The listing builds one solid part. Answer for the finished solid, in the listing's coordinates (mm). Give positions to 0.01 mm unless a question says otherwise; leave off trailing zeros. Order: outer loops, then holes, each group sorted by start corner. A loop starts at its lowest first (then second) coordinate and runs counter-clockwise, first axis right, second up. Notation, with made-up numbers: (1.25, 71) - (54.25, 71) arc R16 cw to (54.25, 85) - close; hole circle Ø2 at (-31, 45.5). An arc over 180 degrees is marked (long way). Answer in a Markdown table with one row per item.
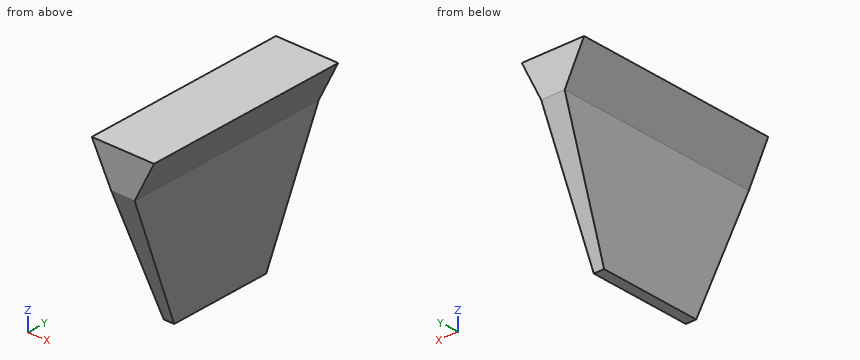
from build123d import *

# Parameters (mm, degrees)
BOSS_EXTRUDE1_DEPTH = 80
SKETCH2_W           = 9.06
SKETCH2_H           = 80
BOSS_EXTRUDE2_DEPTH = 50
CUT_EXTRUDE1_DEPTH  = 105.399039741
CUT_EXTRUDE2_DEPTH  = 106.848049103


with BuildPart() as part:
    # Sketch1 → Boss-Extrude1 (new body)
    with BuildSketch(Plane(origin=(0, 0, 0), x_dir=(1, 0, 0), z_dir=(0, 1, 0))):
        Polygon((-24.06, 0), (-16.56, 14.999429989), (-7.5, 14.999429989), (0, 0), align=None)
    extrude(amount=BOSS_EXTRUDE1_DEPTH)

    # Sketch2 → Boss-Extrude2 (add)
    with BuildSketch(Plane(origin=(0, 0, -14.999429989), x_dir=(-1, 0, 0), z_dir=(0, 0, -1))):
        with Locations((12.03, 40)):
            Rectangle(SKETCH2_W, SKETCH2_H)
    extrude(amount=BOSS_EXTRUDE2_DEPTH)

    # Sketch3 → Cut-Extrude1 (cut, through all)
    with BuildSketch(Plane.ZY.offset(16.56)):
        Polygon((-14.999429989, 80), (-64.999429989, 60), (-64.999429989, 80), align=None)
        Polygon((-64.999429989, 0), (-64.999429989, 20), (-14.999429989, 0), align=None)
    extrude(amount=-CUT_EXTRUDE1_DEPTH, mode=Mode.SUBTRACT)

    # Sketch7 → Cut-Extrude2 (cut, through all)
    with BuildSketch(Plane(origin=(0, 80, 0), x_dir=(1, 0, 0), z_dir=(0, 1, 0))):
        Polygon((-16.56, 14.999429989), (-14.03, 64.999429989), (-16.56, 64.999429989), align=None)
        Polygon((-7.5, 14.999429989), (-7.5, 64.999429989), (-10.03, 64.999429989), align=None)
    extrude(amount=-CUT_EXTRUDE2_DEPTH, mode=Mode.SUBTRACT)


solid = part.part
Item 1: Find section D-D on x = -22. Write down the section's boundary in (y, z).
Answer block:
| item | result |
|---|---|
| outline | (0, -4.12) - (80, -4.12) - (80, 0) - (0, 0) - close |
Item 2: Consider line 1 (Z direction, x = -18, y = 34); line 2 (X direction, y = 38, z = -16); line 3 (X direction, y = 26, z = -37). Determine where each line is inside the solid, lowest interval first.
Answer block:
| item | result |
|---|---|
| line 1 | -12.12 to 0 |
| line 2 | -16.51 to -7.55 |
| line 3 | -15.45 to -8.61 |
Item 3: Find section C-C on x = -8.5. Write down the section's boundary in (y, z), then the cut area to 3 significant figures.
Answer block:
| item | result |
|---|---|
| outline | (0, -15) - (7.91, -34.76) - (72.09, -34.76) - (80, -15) - (80, 0) - (0, 0) - close |
| area | 2,620 mm² |
Item 4: Find section B-B on z = -7.5. Write down the section's boundary in (x, y), then the cut area to 3 significant figures.
Answer block:
| item | result |
|---|---|
| outline | (-20.31, 0) - (-3.75, 0) - (-3.75, 80) - (-20.31, 80) - close |
| area | 1,320 mm² |
Item 5: Find section A-A on y = 39.5. Write down the section's boundary in (x, z).
Answer block:
| item | result |
|---|---|
| outline | (-24.06, 0) - (-16.56, -15) - (-14.03, -65) - (-10.03, -65) - (-7.5, -15) - (0, 0) - close |
Item 6: Each of these flat-tipped pins is pushed along its axis until it touches: P1, Ø1.5, axis at y = 52.5, z = -56, coming from the +X side; P2, Ø3, axis at y = 62.5, z = -22, coming from the -X side; P3, Ø2, axis at y = 36, z = -47, coming from the +X side; P4, Ø6, axis at x = -20, z = -29.5, coming from the +Y side. Where does it stop, or does it pass through?
Answer block:
| item | result |
|---|---|
| P1 | x = -9.54 |
| P2 | x = -16.28 |
| P3 | x = -9.07 |
| P4 | through |
